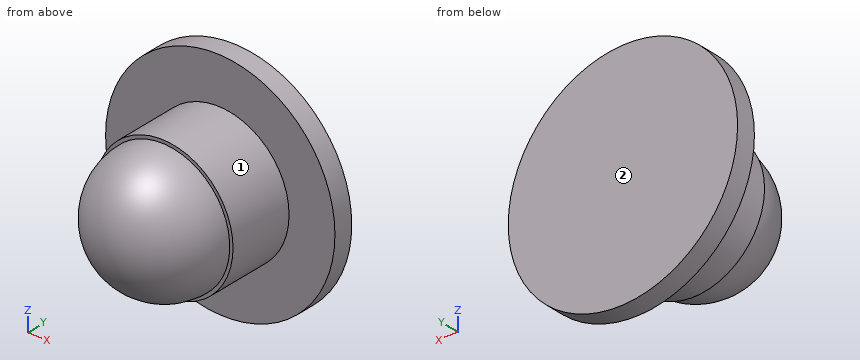
Autodesk Inventor part; units mm, degrees
ref_plane "Work Plane1" through (0, 10, 0) normal (0, 1, 0) x (-1, 0, 0)
ref_plane "YZ Plane" through (0, 0, 0) normal (1, 0, 0) x (0, 1, 0)
ref_plane "XY Plane" through (0, 0, 0) normal (0, 0, 1) x (1, 0, 0)
sketch "Sketch1" plane through (0, 0, 0) normal (0, 1, 0) x (-1, 0, 0)
  arc A0 (0, 10) -> (0, -10) centre (0, 0) ccw
  line L0 (0, 10) -> (0, -10)
  dimension "d0" = 20
revolve "Revolution1" add sketch "Sketch1" angle 360 about axis through (0, 0, 10) along (0, 0, -1)
ref_plane "Work Plane1" through (0, 10, 0) normal (0, 1, 0) x (-1, 0, 0)
sketch "Sketch2" plane through (0, 10, 0) normal (0, 1, 0) x (-1, 0, 0)
  circle A0 centre (0, 0) radius 10.5
  dimension "d2" = 21
sketch "Sketch3" plane through (0, 0, 0) normal (0, 1, 0) x (-1, 0, 0)
  arc A0 (0, 10.5) -> (0, -10.5) centre (0, 0) ccw
  line L0 (0, 10.5) -> (0, -10.5)
  dimension "d3" = 21
revolve "Revolution2" add sketch "Sketch3" angle 180 about axis through (0, 0, 10.5) along (0, 0, 1)
extrude "Extrusion1" add sketch "Sketch2" against normal up to next
sketch "Sketch4" plane through (0, 10, 0) normal (0, 1, 0) x (1, 0, 0)
  circle A0 centre (0, 0) radius 3.2016
  circle A1 centre (0, 0) radius 17.5
  dimension "d7" = 35
extrude "Extrusion2" add sketch "Sketch4" along normal blind 3 contours A0 | A1
properties part number "chasis wheel"
Could you check a few things on this model? Use its own coordinates, in mm. Face numbers are marked on the shaded views. A direction names the side the tool comes from. Coordinates: 2 decimals unless noted, no trailing zeros. Order: outer loops, then holes, each group sorted by start corner. A loop starts at its lowest first (then second) coordinate and runs counter-clockwise, first axis right, second up. Notation, with made-up numbers: M 33,41 L 37,41 A18 ccw 37,60 Z; hole C 35.5,-36.5 d3. An arc over 180 degrees is marked long. Use a Markdown table: item, result. Add a question column.
Q1. I want a section at D-D on z = -12. List the corners of the cut face in (x, y) for me.
Q2. Which directions (+Z, -Z, +X, -X, +Y, -Y) give clear straight access to the entire face, cutting with the end or side of a thin tool? Please do the marked faces 1 and 2.
Q3. If I drill on L1, parallel to Y at x = 7, z = 15.5; L2, parallel to Z at x = 0, y = 6.75; L3, parallel to Z at x = 0, y = 12, over which ranges is the centre line in solid material (lowest first)?
Q4. I'm going to push flat-ended pins straight in: pin 1 (6.5 mm diameter, centred on x = 4, z = -4.5, fed in from -Y); pin 2 (5 mm diameter, centred on x = -3, y = 10.5, fed in from -Z); pin 3 (5 mm diameter, centred on x = 2, y = 4.5, fed in from -Z). Where does each tip first touch, or does it pass through?
Q5. I want a section at C-C on y = 2.75. List the corners of the cut face in (x, z) for me, then the cut area to 3 significant figures.
Q6. I want a section at A-A on x = 0. List the corners of the cut face in (y, z) for me.
Q7. I want a section at B-B on z = 0. List the corners of the cut face in (x, y) for me, then the cut area to 3 significant figures.
Checked values:
| question | item | result |
|---|---|---|
| 1 | outline | M -12.74,10 L 12.74,10 L 12.74,13 L -12.74,13 Z |
| 2 | face 1 | -Y |
| 2 | face 2 | +Z, -Z, +X, -X, +Y |
| 3 | L1 | 10 to 13 |
| 3 | L2 | -10.5 to 10.5 |
| 3 | L3 | -17.5 to 17.5 |
| 4 | pin 1 | y = -9.61 |
| 4 | pin 2 | z = -17.49 |
| 4 | pin 3 | z = -10.5 |
| 5 | outline | C 0,0 d21 |
| 5 | area | 346 mm² |
| 6 | outline | M 0,-10.5 L 10,-10.5 L 10,-17.5 L 13,-17.5 L 13,17.5 L 10,17.5 L 10,10.5 L 0,10.5 L 0,10 A10 ccw 0,-10 Z |
| 7 | outline | M -17.5,10 L -10.5,10 L -10.5,0 L -10,0 A10 ccw 10,0 L 10.5,0 L 10.5,10 L 17.5,10 L 17.5,13 L -17.5,13 Z |
| 7 | area | 472 mm² |
